Job drawing, mm, ordinate dimensions from the low corner. One solid piece. Coordinates: 2 decimals unless noted, no trailing zeros. Write each loop counter-clockwise with the first axis right and the second up, starting at its lowest first coordinate (ties: lowest second). Pieces come first, ordered by that corner, then holes.
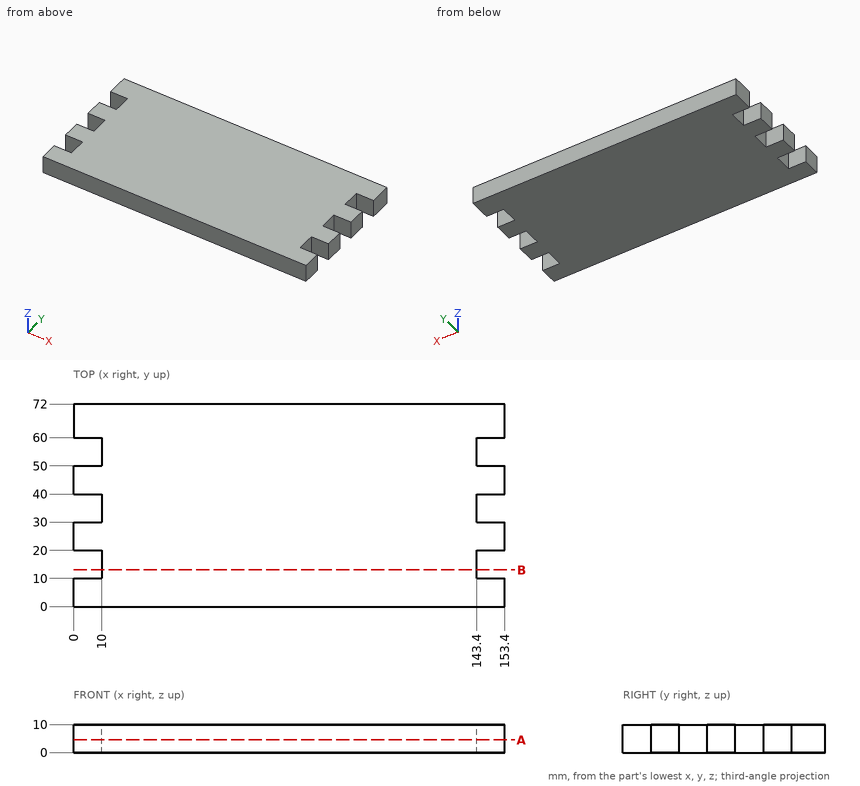
1. Probe line 1 along Y through (x, z) = (144, 3.25); line 2 along X through (y, z) = (57, 2). List the from-to ranges inside material, lowest first.
Computed values:
line 1: y = 0 to 10, 20 to 30, 40 to 50, 60 to 72
line 2: x = 10 to 143.4
2. Saw through at B-B on y = 13. List the corners of the cut face in (x, z).
Computed values:
outline: (10, 0) - (143.4, 0) - (143.4, 10) - (10, 10) - close
3. Saw through at A-A on z = 4.5. List the corners of the cut face in (x, y), plus the area to 3 significant figures.
Computed values:
outline: (0, 0) - (153.4, 0) - (153.4, 10) - (143.4, 10) - (143.4, 20) - (153.4, 20) - (153.4, 30) - (143.4, 30) - (143.4, 40) - (153.4, 40) - (153.4, 50) - (143.4, 50) - (143.4, 60) - (153.4, 60) - (153.4, 72) - (0, 72) - (0, 60) - (10, 60) - (10, 50) - (0, 50) - (0, 40) - (10, 40) - (10, 30) - (0, 30) - (0, 20) - (10, 20) - (10, 10) - (0, 10) - close
area: 10,400 mm2
4. Flat gauge pins, fed straight in: pin 1 (3 mm diameter, centred on y = 15.5, z = 6, fed in from +X); pin 2 (5 mm diameter, centred on y = 16.5, z = 6, fed in from -X). Where does each tip first touch, or does it go through?
Computed values:
pin 1: stops at x = 143.4
pin 2: stops at x = 10
